The model under review builds one solid part; all positions refer to its coordinate system, in mm. A direction names the side the tool comes from. Give positions to 0.01 mm unless a question says otherwise; leave off trailing zeros. Order: outer loops, then holes, each group sorted by start corner. A loop starts at its lowest first (then second) coordinate and runs counter-clockwise, first axis right, second up. Notation, with made-up numbers: (60.5, 67.25) - (119.5, 67.25) arc R17 ccw to (119.5, 93.25) - close; hole circle Ø3 at (86.25, -12). An arc over 180 degrees is marked (long way). Use CSV: the item, a comma, the result in double quotes.
```python
from build123d import *

# Parameters (mm, degrees)
F0_W     = 13.4990522638
F0_H     = 6.7189366567
F0_H_2   = 5.0193380237
F1_DEPTH = 25.4


with BuildPart() as f1:
    # F0 (on Top) → F1 (new body)
    with BuildSketch(Plane.XY):
        with Locations((-14.9052026682, 36.7298916125)):
            Rectangle(F0_W, F0_H)
        Polygon((-49.1617234445, 24.0451842546), (-46.0720470312, 28.3510852605), (-69.4638639688, 28.3510852605), (-69.4638639688, 20.6704232842), (-64.4017234445, 24.0451842546), align=None)
        Polygon((-18.5611955822, -44.5749908686), (-5.08, 19.6878403194), (-10.16, 19.6878403194), (-31.7790172994, -44.5749908686), align=None)
        Polygon((21.9359565526, -45.1374538243), (0, 19.6878403194), (-5.08, 19.6878403194), (7.3119853623, -44.5749908686), align=None)
        with Locations((-14.9052026682, 30.8607542723)):
            Rectangle(F0_W, F0_H_2)
        with BuildLine():
            Line((-41.9020165778, 22.7089282594), (-44.6144271886, 19.7146166008))
            add(Edge.make_bspline(
                [(-31.2667824328, 24.3264157325), (-31.9929960152, 21.6699538462), (-34.7602014448, 18.1939718361), (-41.4758034197, 18.5698095031), (-44.6144271886, 19.7146166008)],
                knots=[0, 0, 0, 0, 0.4544832874, 1, 1, 1, 1], degree=3))
            Line((-31.2667824328, 24.3264157325), (-37.5335417804, 24.3264157325))
            add(Edge.make_bspline(
                [(-37.5335417804, 24.3264157325), (-36.8480037486, 22.5468860707), (-34.5986306719, 21.0862357426), (-37.8524884582, 21.3479679078), (-41.9020165778, 22.7089282594)],
                knots=[0, 0, 0, 0, 0.4183773916, 1, 1, 1, 1], degree=3))
        make_face()
        Polygon((0, 19.6878403194), (0, 24.3264157325), (-10.16, 24.3264157325), (-10.16, 19.6878403194), (-5.08, 19.6878403194), align=None)
        with BuildLine():
            Line((-8.1556765363, 28.3510852605), (-21.6547288001, 28.3510852605))
            Line((-21.6547288001, 28.3510852605), (-46.0720470312, 28.3510852605))
            Line((-46.0720470312, 28.3510852605), (-49.1617234445, 24.0451842546))
            Line((-49.1617234445, 24.0451842546), (-55.57827127, 15.1028174692))
            Line((-55.57827127, 15.1028174692), (-48.7920460626, 15.1028174692))
            Line((-48.7920460626, 15.1028174692), (-44.6144271886, 19.7146166008))
            Line((-44.6144271886, 19.7146166008), (-41.9020165778, 22.7089282594))
            Line((-41.9020165778, 22.7089282594), (-40.4368083146, 24.3264157325))
            Line((-40.4368083146, 24.3264157325), (-37.5335417804, 24.3264157325))
            Line((-37.5335417804, 24.3264157325), (-31.2667824328, 24.3264157325))
            Line((-31.2667824328, 24.3264157325), (-10.16, 24.3264157325))
            Line((-10.16, 24.3264157325), (0, 24.3264157325))
            Line((0, 24.3264157325), (67.6737308797, 24.5399160971))
            ThreePointArc((67.6737308797, 24.5399160971), (66.0991955865, 26.6047667833), (68.04705303, 28.3219217342))
            Line((68.04705303, 28.3219217342), (68.0443234637, 28.3510852605))
            Line((68.0443234637, 28.3510852605), (-8.1556765363, 28.3510852605))
        make_face()
        with BuildLine():
            Line((-40.4368083146, 24.3264157325), (-41.9020165778, 22.7089282594))
            add(Edge.make_bspline(
                [(-37.5335417804, 24.3264157325), (-36.8480037486, 22.5468860707), (-34.5986306719, 21.0862357426), (-37.8524884582, 21.3479679078), (-41.9020165778, 22.7089282594)],
                knots=[0, 0, 0, 0, 0.4183773916, 1, 1, 1, 1], degree=3))
            Line((-37.5335417804, 24.3264157325), (-40.4368083146, 24.3264157325))
        make_face()
        with BuildLine():
            ThreePointArc((69.8999820042, 26.4176335186), (69.3603061972, 27.7461344963), (68.04705303, 28.3219217342))
            ThreePointArc((68.04705303, 28.3219217342), (66.0991955865, 26.6047667833), (67.6737308797, 24.5399160971))
            Line((67.6737308797, 24.5399160971), (68.0443234637, 24.5410852605))
            Line((68.0443234637, 24.5410852605), (68.0443234637, 24.5132726231))
            ThreePointArc((68.0443234637, 24.5132726231), (69.3593537425, 25.0881543876), (69.8999820042, 26.4176335186))
        make_face()
        with BuildLine():
            Line((68.0443234637, 24.5410852605), (67.6737308797, 24.5399160971))
            ThreePointArc((67.6737308797, 24.5399160971), (67.8583760557, 24.5175377802), (68.0443234637, 24.5132726231))
            Line((68.0443234637, 24.5132726231), (68.0443234637, 24.5410852605))
        make_face()
    extrude(amount=F1_DEPTH)


solid = f1.part
```
Item 1: Take a section at B-B, the plane x = -51. Give the boundary of the cut face in (y, z), and give its area (3 significant figures).
Results list:
outline,"(15.1, 0) - (21.48, 0) - (21.48, 25.4) - (15.1, 25.4) - close; (24.05, 0) - (28.35, 0) - (28.35, 25.4) - (24.05, 25.4) - close"
area,"271 mm2"
Item 2: Mouldability with a two-part tool opening along Y and no side actions: class faces 1 (the face through (11.12, -13.18, 12.52)), 2 (the face through (30, 28.351, 13)), 3 (the face through (-10, 1, 0)), 4 (the face through (-66.968, 22.334, 12.522)) as pulls with the +Y half, pulls with the -Y half, needs draft (parallel to the pull), parting line crosses it, or undercut.
Results list:
face 1,"undercut"
face 2,"pulls with the +Y half"
face 3,"needs draft"
face 4,"pulls with the -Y half"
Item 3: Take a section at C-C, the plane y = 30.5. Give the boundary of the cut face in (x, z), and give its area (3 significant figures).
Results list:
outline,"(-21.65, 0) - (-8.16, 0) - (-8.16, 25.4) - (-21.65, 25.4) - close"
area,"343 mm2"
Item 4: Clearance check with flat-ended pins moving along their axes: pin 1 (9.5 mm diameter, centred on y = 35.5, z = 12, fed in from -X); pin 2 (6 mm diameter, centred on x = 51, z = 16, fed in from -Y); pin 3 (7.5 mm diameter, centred on x = 44.5, z = 18, fed in from +Y). State where each tip first meets the part, or that it passes through.
Results list:
pin 1,"stops at x = -21.65"
pin 2,"stops at y = 24.48"
pin 3,"stops at y = 28.35"
Item 5: Take a section at D-D, the plane x = 43.5. Give the boundary of the cut face in (y, z).
Results list:
outline,"(24.46, 0) - (28.35, 0) - (28.35, 25.4) - (24.46, 25.4) - close"
Item 6: Wall thickness on L1, parallel to X at y = 23, z = 16; L2, parallel to X at y = 24, z = 23; L3, parallel to X at y = 20.5, z = 21: over which ranges is each line inside the solid? List them lowest first.
Results list:
L1,"x = -69.46 to -65.97, -49.91 to -31.71, -10.16 to 0"
L2,"x = -69.46 to -64.47, -49.19 to -31.36, -10.16 to 0"
L3,"x = -51.71 to -33.36, -10.16 to 0"
Item 7: Tool access review of faces 5 (the face through (0, 22, 13)), 6 (the face through (-21.655, 34, 13)), 7 (the face through (-11.915, -12.893, 12.522)): name each direction out of +Z, -Z, +X, -X, +Y, -Y from which nothing blocks a thin tool from reaching the whole face with its end or side.
Results list:
face 5,"+Z, -Z, +X"
face 6,"+Z, -Z, -X, +Y"
face 7,"+Z, -Z, -Y"
Item 8: Take a section at A-A, the plane y = 2.5. Give the boundary of the cut face in (x, z).
Results list:
outline,"(-15.94, 0) - (-8.69, 0) - (-8.69, 25.4) - (-15.94, 25.4) - close; (-1.77, 0) - (5.82, 0) - (5.82, 25.4) - (-1.77, 25.4) - close"
